Model file for the job. Use its own axes, mm. Coordinates: 2 decimals unless noted, no trailing zeros. Return JSON: item names as keys, results as strings. Group by question number.
1) Pull direction Y, two halves, no side cores. Call faces 1 (the cylindrical face through (-12.44, -130.14, -0.54)), 2 (the cylindrical face through (-9.86, 139.237, 3.83)), 3 (the cylindrical face through (-9.86, -120.763, 3.83)): +Y half, -Y half, draft (parallel to the pull), parting line (faces both ways), or undercut.
2) Flat gauge pins, fed straight in: pin 1 (10 mm diameter, centred on y = 55.5, z = 0, fed in from +X); pin 2 (1 mm diameter, centred on x = 66, z = 7.5, fed in from +Y); pin 3 (5 mm diameter, centred on y = -18, z = -3, fed in from -X). Where does each tip first touch, or does it go through?
3) Probe line 1 (Y direction, x = 16.5, z = -2); line 2 (Z direction, x = -10, y = -130.75); line 3 (Z direction, x = -10, y = -125.5). List the from-to ranges inside material, lowest first.
from build123d import *

# Parameters (mm, degrees)
BALAYAGE2_PROFILE_R          = 10
ESQUISSE38_R                 = 10
BOSS_EXTRU_1_DEPTH           = 20
ESQUISSE39_R                 = 10
BOSS_EXTRU_2_DEPTH           = 20
ENL_V_MAT_EXTRU_1_DEPTH      = 199.242276162
ENL_V_MAT_EXTRU_1_DEPTH_BACK = 199.242276162
ESQUISSE41_R                 = 2.5


with BuildPart() as part:
    # Balayage2: sweep along a path in Esquisse2
    with BuildLine(Plane.XY) as balayage2_path:
        ThreePointArc((0, -130), (130, 0), (0, 130))
    # Balayage2 profile (on start of the path) → Balayage2 (sweep)
    with BuildSketch(Plane(origin=(0, -130, 0), x_dir=(0, 1, 0), z_dir=(1, 0, 0))):
        Circle(BALAYAGE2_PROFILE_R)
    sweep(path=balayage2_path.line)

    # Esquisse38 → Boss.-Extru.1 (add)
    with BuildSketch(Plane.ZY):
        with Locations(Location((0, -130, 0), (0, 0, 90))):
            Circle(ESQUISSE38_R)
    extrude(amount=BOSS_EXTRU_1_DEPTH)

    # Esquisse39 → Boss.-Extru.2 (add)
    with BuildSketch(Plane.ZY):
        with Locations(Location((0, 130, 0), (0, 0, 90))):
            Circle(ESQUISSE39_R)
    extrude(amount=BOSS_EXTRU_2_DEPTH)

    # Esquisse41 → Enlèv. mat.-Extru.1 (cut, two sides: drawn at the far end of the back side and taken through both)
    with BuildSketch(Plane(origin=(0, 0, 0), x_dir=(1, 0, 0), z_dir=(0, 1, 0)).offset(-ENL_V_MAT_EXTRU_1_DEPTH_BACK)):
        with Locations(Location((-10, 0, 0), (0, 0, 270))):
            Circle(ESQUISSE41_R)
    extrude(amount=ENL_V_MAT_EXTRU_1_DEPTH + ENL_V_MAT_EXTRU_1_DEPTH_BACK, mode=Mode.SUBTRACT)


solid = part.part
Answers below:
{
 "1": {"face 1": "draft", "face 2": "undercut", "face 3": "undercut"},
 "2": {"pin 1": "stops at x = 130.57", "pin 2": "stops at y = 120.28", "pin 3": "stops at x = 118.43"},
 "3": {"line 1": "y = -138.82 to -119.06, 119.06 to 138.82", "line 2": "z = -9.97 to -2.5, 2.5 to 9.97", "line 3": "z = -8.93 to -2.5, 2.5 to 8.93"}
}
